```python
from build123d import *

# Parameters (mm, degrees)
F1_DEPTH      = 31.75
F1_DEPTH_BACK = 12.7
F2_R          = 3.175
F3_DEPTH      = 25.4
F4_R          = 1.5875
F5_DEPTH      = 25.4
F7_DEPTH      = 25.4
F8_R          = 5.08


with BuildPart() as f1:
    # F0 (on Front) → F1 (new body, two sides)
    with BuildSketch(Plane.XZ) as f1_sk:
        Polygon((-37.854384, 0), (0, 0), (37.854384, 0), (37.854384, 35.133872), (19.893872, 53.094384), (0, 53.094384), (-19.893872, 53.094384), (-37.854384, 35.133872), align=None)
    extrude(amount=F1_DEPTH)
    extrude(f1_sk.sketch, amount=-F1_DEPTH_BACK)

    # F2 (on face) → F3 (cut)
    with BuildSketch(Plane(origin=(-36.494128, 0, 36.494128), x_dir=(0, -1, 0), z_dir=(-0.707107, 0, 0.707107))):
        with Locations((0, 10.776307)):
            Circle(F2_R)
    extrude(amount=-F3_DEPTH, mode=Mode.SUBTRACT)

    # F4 (on face) → F5 (cut)
    with BuildSketch(Plane(origin=(36.494128, 0, 36.494128), x_dir=(0.707107, 0, -0.707107), z_dir=(0.707107, 0, 0.707107))):
        with Locations((-10.776307, 0)):
            Circle(F4_R)
    extrude(amount=-F5_DEPTH, mode=Mode.SUBTRACT)

    # F6 (on face) → F7 (cut)
    with BuildSketch(Plane.XZ.offset(31.75)):
        with BuildLine():
            Line((0, 24.220256), (-4.490128, 19.730128))
            ThreePointArc((-4.490128, 19.730128), (0, 8.89), (4.490128, 19.730128))
            Line((4.490128, 19.730128), (0, 24.220256))
        make_face()
    extrude(amount=-F7_DEPTH, mode=Mode.SUBTRACT)

    # F8
    f8_edges = [f1.edges().sort_by_distance(p)[0] for p in [
        (-37.854384, 12.7, 17.566936),
        (-28.874128, 12.7, 44.114128),
        (0, 12.7, 53.094384),
        (28.874128, 12.7, 44.114128),
        (37.854384, 12.7, 17.566936),
        (-19.893872, -9.525, 53.094384),
        (-37.854384, -9.525, 35.133872),
        (-28.874128, -31.75, 44.114128),
        (-37.854384, -31.75, 17.566936),
        (0, -31.75, 53.094384),
        (19.893872, -9.525, 53.094384),
        (28.874128, -31.75, 44.114128),
        (37.854384, -31.75, 17.566936),
        (37.854384, -9.525, 35.133872),
    ]]
    fillet(f8_edges, radius=F8_R)


solid = f1.part
```
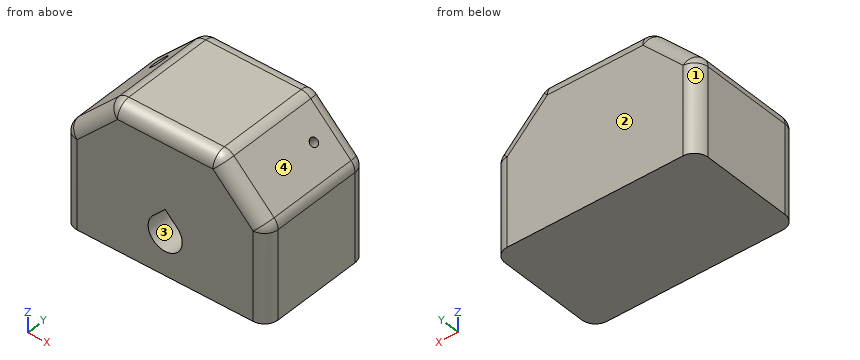
Model file for the job. Use its own axes, mm. Face numbers are marked on the shaded views. Coordinates: 2 decimals unless noted, no trailing zeros. Order: outer loops, then holes, each group sorted by start corner. A loop starts at its lowest first (then second) coordinate and runs counter-clockwise, first axis right, second up. Notation, with made-up numbers: (47, 57.5) -> (97, 57.5) arc R21 ccw to (97, 88.5) -> close; hole circle Ø8 at (87, 73). An arc over 180 degrees is marked (long way). Answer as a JSON object with one key per item and string values. Group by question number.
1) Cut at C-C, the plane y = 9.5. Write the cut outline in (x, z), then the cut area to 3 significant figures.
2) Drill centre lines: L1, parallel to X at y = -23, z = 15; L2, parallel to X at y = 8, z = 23; L3, parallel to X at y = -8.5, z = 17. Where is each one in solid material? Low to high.
3) Pull direction X, two halves, no side cores. Call the marked faces 1, 2, 3 and 4: +X half, -X half, draft (parallel to the pull), parting line (faces both ways), or undercut.
4) Cut at B-B, the plane z = 15.24. Write the cut outline in (x, y).
5) Cut at D-D, the plane z = 21.5. Write the cut outline in (x, y), then the cut area to 3 significant figures.
6) Flat gauge pin, fed straight in: pin 1 (11.5 mm diameter, centred on x = 0, z = 15.24, fed in from -Y). Where does the tip first touch, or does it go through?
7) Cut at A-A, the plane y = -15.5. Write the cut outline in (x, z).
Check values:
{
 "1": {"outline": "(-37.49, 0) -> (37.49, 0) -> (37.49, 33.03) arc R4.72 ccw to (36.11, 36.37) -> (21.13, 51.35) arc R4.72 ccw to (17.79, 52.73) -> (-17.79, 52.73) arc R4.72 ccw to (-21.13, 51.35) -> (-36.11, 36.37) arc R4.72 ccw to (-37.49, 33.03) -> close", "area": "3,640 mm²"},
 "2": {"L1": "x = -37.85 to -6.35, 6.35 to 37.85", "L2": "x = -37.84 to 37.84", "L3": "x = -37.85 to -6.1, 6.1 to 37.85"},
 "3": {"face 1": "-X half", "face 2": "draft", "face 3": "undercut", "face 4": "+X half"},
 "4": {"outline": "(-37.85, -26.67) arc R5.08 ccw to (-32.77, -31.75) -> (-6.35, -31.75) -> (-6.35, -6.35) -> (6.35, -6.35) -> (6.35, -31.75) -> (32.77, -31.75) arc R5.08 ccw to (37.85, -26.67) -> (37.85, 7.62) arc R5.08 ccw to (32.77, 12.7) -> (-32.77, 12.7) arc R5.08 ccw to (-37.85, 7.62) -> close"},
 "5": {"outline": "(-37.85, -26.67) arc R5.08 ccw to (-32.77, -31.75) -> (-2.72, -31.75) -> (-2.72, -6.35) -> (2.72, -6.35) -> (2.72, -31.75) -> (32.77, -31.75) arc R5.08 ccw to (37.85, -26.67) -> (37.85, 7.62) arc R5.08 ccw to (32.77, 12.7) -> (-32.77, 12.7) arc R5.08 ccw to (-37.85, 7.62) -> close", "area": "3,200 mm²"},
 "6": {"pin 1": "stops at y = -6.35"},
 "7": {"outline": "(-37.85, 0) -> (37.85, 0) -> (37.85, 33.03) arc R5.08 ccw to (36.37, 36.62) -> (21.38, 51.61) arc R5.08 ccw to (17.79, 53.09) -> (-17.79, 53.09) arc R5.08 ccw to (-21.38, 51.61) -> (-36.37, 36.62) arc R5.08 ccw to (-37.85, 33.03) -> close; hole (-4.49, 19.73) arc R6.35 ccw (long way) to (4.49, 19.73) -> (0, 24.22) -> close"}
}
